Autodesk Inventor part; units mm, degrees
ref_plane "YZ Plane" through (0, 0, 0) normal (1, 0, 0) x (0, 1, 0)
ref_plane "XZ Plane" through (0, 0, 0) normal (0, 1, 0) x (-1, 0, 0)
ref_plane "XY Plane" through (0, 0, 0) normal (0, 0, 1) x (1, 0, 0)
sketch "Skizze4" plane through (0, 0, 0) normal (0, 1, 0) x (-1, 0, 0)
  arc A0 (3, 0) -> (-3, 0) centre (0, 0) ccw
  line L0 (3, 0) -> (3, -4)
  line L1 (3, -4) -> (-3, -4) construction
  line L2 (-3, -4) -> (-3, 0)
  line L3 (29.4604, -19.0022) -> (26.5011, -24.2217) construction
  line L4 (26.5011, -24.2217) -> (6.9282, -13.1244) construction
  arc A1 (26.5011, -24.2217) -> (29.4604, -19.0022) centre (27.9808, -21.612) ccw construction
  line L5 (0, 0) -> (3, -1.7009) construction
  line L6 (-2.4661, -4.3495) -> (27.9808, -21.612) construction
  line L7 (27.9808, -21.612) -> (30.4468, -17.2624) construction
  line L8 (30.4468, -17.2624) -> (0, 0) construction
  line L9 (0, 0) -> (-2.4661, -4.3495) construction
  line L10 (-2.4661, -4.3495) -> (30.4468, -17.2624) construction
  line L11 (27.9808, -21.612) -> (0, 0) construction
  line L12 (9.8874, -7.905) -> (29.4604, -19.0022) construction
  line L13 (6.9282, -13.1244) -> (0.0407, -9.2195)
  line L14 (9.8874, -7.905) -> (6.9282, -13.1244)
  line L15 (9.8874, -7.905) -> (3, -4)
  arc A2 (-3, -4) -> (0.0407, -9.2195) centre (3, -4) ccw
  point P0 (13.9904, -10.806)
  dimension "d15" = 4
  dimension "d16" = 3
  dimension "d17" = 5
  dimension "d18" = 35
  dimension "d19" = 5
extrude "Extrusion4" add sketch "Skizze4" along normal blind 5
sketch "Skizze5" plane through (0, 0, 0) normal (0, -1, 0) x (1, 0, 0)
  line L0 (-9.8874, -7.905) -> (-29.4604, -19.0022) construction
  line L1 (-26.5011, -24.2217) -> (-6.9282, -13.1244) construction
  line L2 (-9.8874, -7.905) -> (-6.9282, -13.1244)
  line L3 (-15.6273, -18.0565) -> (-6.9282, -13.1244)
  line L4 (-6.9282, -13.1244) -> (-9.8874, -7.905)
  line L5 (-9.8874, -7.905) -> (-18.5865, -12.8371)
  line L6 (-18.5865, -12.8371) -> (-15.6273, -18.0565)
  line L7 (-15.6273, -18.0565) -> (-9.8874, -7.905) construction
  line L8 (-6.9282, -13.1244) -> (-18.5865, -12.8371) construction
  line L9 (-14.237, -10.371) -> (-11.2777, -15.5905) construction
  point P0 (0, 0)
  point P1 (-13.9904, -10.806)
  point P2 (-12.7573, -12.9808)
  point P3 (-12.7573, -12.9808)
extrude "Extrusion5" add sketch "Skizze5" along normal mid plane 10
sketch "Skizze6" plane through (0, -5, 0) normal (0, -1, 0) x (1, 0, 0)
  line L0 (-9.8874, -7.905) -> (-29.4604, -19.0022) construction
  arc A0 (-26.5011, -24.2217) -> (-29.4604, -19.0022) centre (-27.9808, -21.612) ccw construction
  line L1 (-26.5011, -24.2217) -> (-6.9282, -13.1244) construction
  line L2 (-18.5865, -12.8371) -> (-15.6273, -18.0565)
  line L3 (-25.8727, -16.9681) -> (-18.5865, -12.8371)
  line L4 (-15.6273, -18.0565) -> (-22.9134, -22.1876)
  arc A1 (-25.8727, -16.9681) -> (-28.9104, -21.9956) centre (-22.9134, -22.1876) ccw
  line L5 (-27.9808, -21.612) -> (-26.0079, -25.0916) construction
  arc A2 (-29.0064, -24.9956) -> (-23.0094, -25.1876) centre (-26.0079, -25.0916) ccw
  line L6 (-28.9104, -21.9956) -> (-29.0064, -24.9956)
  line L7 (-23.0094, -25.1876) -> (-22.9134, -22.1876)
  point P0 (0, 0)
  dimension "d45" = 4
  dimension "d46" = 3
extrude "Extrusion6" add sketch "Skizze6" against normal blind 5
sketch "Skizze7" plane through (0, 0, 0) normal (0, -1, 0) x (1, 0, 0)
  circle A0 centre (0, 0) radius 1.05
  dimension "d26" = 2.1
extrude "Extrusion7" cut sketch "Skizze7" against normal up to next
sketch "Skizze8" plane through (0, -5, 0) normal (0, -1, 0) x (1, 0, 0)
  arc A0 (-29.0064, -24.9956) -> (-23.0094, -25.1876) centre (-26.0079, -25.0916) ccw construction
  circle A1 centre (-26.0079, -25.0916) radius 1.05
  point P0 (0, 0)
  dimension "d47" = 2.1
extrude "Extrusion8" cut sketch "Skizze8" against normal up to next
chamfer "Fase2" distance 9 distance2 5 1 edges at (-17.1069, 5, -15.4468) measured on face at (-7.2091, 5, -8.6855)
chamfer "Fase3" distance 9 distance2 5 1 edges at (-8.4078, -5, -10.5147) measured on face at (-19.5579, -5, -15.6869)
fillet "Rundung2" [suppressed]
properties part number "LegConnector" material "ABS-Kunststoff"
Geometry check sheet. Reference: the model listing, model coordinates, mm. A direction names the side the tool comes from. Round coordinates to 2 decimals unless told otherwise and drop trailing zeros. Write each loop counter-clockwise with the first axis right and the second up, starting at its lowest first coordinate (ties: lowest second). Pieces come first, ordered by that corner, then holes. Notation, with made-up numbers: (66, -20.5) - (102, -20.5) arc R17 ccw to (102, 7.5) - close; hole circle Ø10 at (73, 50). An arc over 180 degrees is marked (long way). Write each question's results on one line, items separated by ' | '.
(1) Depth check by flat-ended pin: pin 1 Ø10.5 at (x, z) = (-6, -3.5) entering from -Y; pin 2 Ø2 at (x, z) = (-21.5, -11.5) entering from -Y; pin 3 Ø2 at (x, z) = (-11.5, -12.5) entering from -Y; pin 4 Ø3 at (y, z) = (-3.5, -19) entering from -X. Enter the tip coordinate at first touch or a pass-through.
Computed:
pin 1: stops at y = 0 | pin 2: passes through | pin 3: stops at y = -2.59 | pin 4: stops at x = -28.67
(2) Set-up check for faces 4 (the face through (-3, 2, -2)), 5 (the face through (-13.227, 2.465, -13.295)): record each of +Z, -Z, +X, -X, +Y, -Y from which the full face is reachable in a straight line by a thin tool's end or side.
Computed:
face 4: +Z, -X, +Y, -Y | face 5: -Z, -X, +Y
(3) Draft check along X on faces 1 (the face through (-26.8, -2.5, -24.4)), 2 (the face through (-26.17, -2.535, -28.087)), 3 (the face through (-28.03, -2.54, -19.05)). Enter one of: pulls with the +X half, pulls with the -X half, needs draft (parallel to the pull), parting line crosses it, or undercut.
Computed:
face 1: undercut | face 2: parting line crosses it | face 3: pulls with the -X half
(4) Sectioned sample at C-C, the plane y = -0.75. Enter the section's corners in (x, z).
Computed:
outline: (-29.01, -25) arc R3 ccw to (-23.01, -25.19) - (-22.91, -22.19) - (-15.63, -18.06) - (-8.1, -13.79) - (-11.06, -8.57) - (-18.59, -12.84) - (-25.87, -16.97) arc R6 ccw to (-28.91, -22) - close; hole circle Ø2.1 at (-26.01, -25.09)
(5) Thickness scan on probe 1 along Y at (x, z) = (-22, -20); probe 2 along X at (y, z) = (-2, -25); probe 3 along Y at (x, z) = (-7.5, -10.5). Record the ranges inside material, lowest first. Write a range as from..to.
Computed:
probe 1: y = -5..0 | probe 2: x = -29.01..-27.05, -24.96..-23 | probe 3: y = 0..5
(6) Sectioned sample at D-D, the plane x = -21. Enter the section's corners in (y, z), plus the area to 3 significant figures.
Computed:
outline: (-5, -21.1) - (0, -21.1) - (0, -14.21) - (-5, -14.21) - close | area: 34.5 mm^2
(7) Sectioned sample at A-A, the plane y = -2.75. Enter the section's corners in (x, z).
Computed:
outline: (-29.01, -25) arc R3 ccw to (-23.01, -25.19) - (-22.91, -22.19) - (-15.63, -18.06) - (-11.23, -15.57) - (-14.19, -10.35) - (-18.59, -12.84) - (-25.87, -16.97) arc R6 ccw to (-28.91, -22) - close; hole circle Ø2.1 at (-26.01, -25.09)
